Source: CAD feature listing. Evaluate the final solid. Frame: model axes, mm. Coordinates: 2 decimals unless noted, no trailing zeros. One line per question, with ' | ' between items. Start each with the question number.
Q1. Cut plane A-A, the plane z = 152.5. Give the number of separate pieces and of enclosed holes in the cut face, plus the area to 3 significant figures.
Q2. Contact query for flat-ended pins moving along their axis: P1, Ø1.5, axis at x = 4, z = 468.5, coming from the -Y side; P2, Ø1.2, axis at y = 5, z = 532, coming from the +X side; P3, Ø0.8, axis at x = -5.5, z = 446.5, coming from the -Y side; P4, Ø6.5, axis at x = 0, y = 0, coming from the +Z side. Output: stop coordinate, or through.
Q3. Line query: line 1 (X direction, y = -14.5, z = 212); line 2 (Y direction, x = -16, z = 647.5); line 3 (X direction, y = 0.5, z = 396.5). Output: solid intervals per line, ascending.
```python
from build123d import *

# Parameters (mm, degrees)
CROQUIS1_W              = 40
CROQUIS1_H              = 40
SALIENTE_EXTRUIR1_DEPTH = 924.8
CROQUIS2_W              = 6
CROQUIS2_H              = 6
CROQUIS2_R              = 3.5
CORTAR_EXTRUIR2_DEPTH   = 924.8
REDONDEO1_R             = 2
REDONDEO2_R             = 2


with BuildPart() as part:
    # Croquis1 → Saliente-Extruir1 (new body)
    with BuildSketch(Plane.XY):
        Rectangle(CROQUIS1_W, CROQUIS1_H)
    extrude(amount=SALIENTE_EXTRUIR1_DEPTH)

    # Croquis2 → Cortar-Extruir2 (cut)
    with BuildSketch(Plane.XY.offset(924.8)):
        with Locations((-15.5, 15.5)):
            Rectangle(CROQUIS2_W, CROQUIS2_H)
        Polygon((4.5, 15.5), (4.5, 20), (-4.5, 20), (-4.5, 15.5), (-7, 15.5), (-7, 18), (-11, 18), (-11, 12.767766953), (-5.733637236, 7.501404189), (5.733637236, 7.501404189), (11, 12.767766953), (11, 18), (7, 18), (7, 15.5), align=None)
        with Locations((15.5, 15.5)):
            Rectangle(CROQUIS2_W, CROQUIS2_H)
        Polygon((15.367588592, -4.5), (20, -4.5), (20, 4.5), (15.367588592, 4.5), (15.367588592, 7), (17.867588592, 7), (17.867588592, 11), (12.767766953, 11), (7.501349817, 5.733582864), (7.501349817, -5.733582864), (12.767766953, -11), (17.867588592, -11), (17.867588592, -7), (15.367588592, -7), align=None)
        Polygon((-20, 4.5), (-20, -4.5), (-15.367588592, -4.5), (-15.367588592, -7), (-17.867588592, -7), (-17.867588592, -11), (-12.767766953, -11), (-7.501349817, -5.733582864), (-7.501349817, 5.733582864), (-12.767766953, 11), (-17.867588592, 11), (-17.867588592, 7), (-15.367588592, 7), (-15.367588592, 4.5), align=None)
        Circle(CROQUIS2_R)
        Polygon((11, -12.767766953), (5.733637236, -7.501404189), (-5.733637236, -7.501404189), (-11, -12.767766953), (-11, -18), (-7, -18), (-7, -15.5), (-4.5, -15.5), (-4.5, -20), (4.5, -20), (4.5, -15.5), (7, -15.5), (7, -18), (11, -18), align=None)
        with Locations((-15.5, -15.5)):
            Rectangle(CROQUIS2_W, CROQUIS2_H)
        with Locations((15.5, -15.5)):
            Rectangle(CROQUIS2_W, CROQUIS2_H)
    extrude(amount=-CORTAR_EXTRUIR2_DEPTH, mode=Mode.SUBTRACT)

    # Redondeo1
    redondeo1_edges = [part.edges().sort_by_distance(p)[0] for p in [
        (20, -20, 462.4),
        (-20, -20, 462.4),
        (-20, 20, 462.4),
        (20, 20, 462.4),
    ]]
    fillet(redondeo1_edges, radius=REDONDEO1_R)

    # Redondeo2
    redondeo2_edges = [part.edges().sort_by_distance(p)[0] for p in [
        (4.5, 20, 462.4),
        (-4.5, 20, 462.4),
        (20, -4.5, 462.4),
        (20, 4.5, 462.4),
        (-20, 4.5, 462.4),
        (-20, -4.5, 462.4),
        (-4.5, -20, 462.4),
        (4.5, -20, 462.4),
    ]]
    fillet(redondeo2_edges, radius=REDONDEO2_R)


solid = part.part
```
Reply:
1) separate pieces: 1 | enclosed holes: 5 | area: 576 mm^2
2) P1: stops at y = -18.97 | P2: stops at x = 19.79 | P3: stops at y = -19.91 | P4: passes through
3) line 1: x = -20 to -18.5, -12.5 to -11, 11 to 12.5, 18.5 to 20 | line 2: y = -20 to -18.5, -12.5 to -11, -7 to -4.5, 4.5 to 7, 11 to 12.5, 18.5 to 20 | line 3: x = -7.5 to -3.46, 3.46 to 7.5
